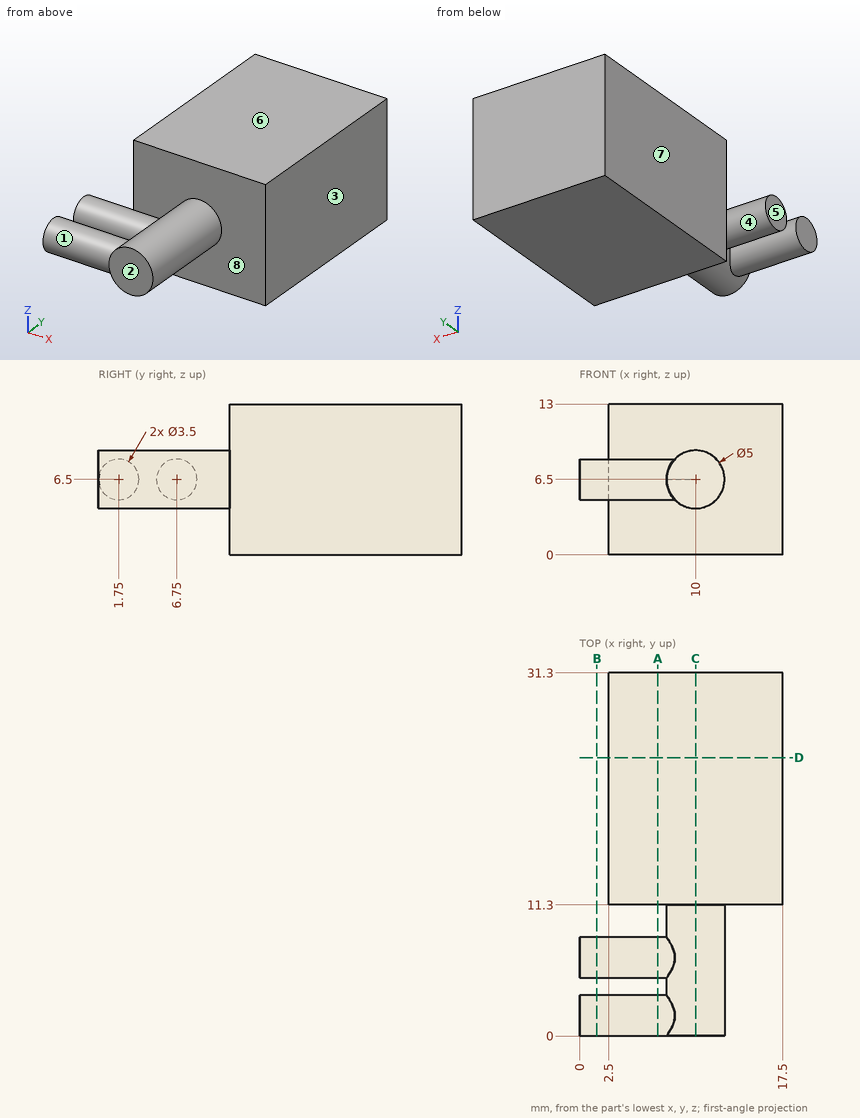
Check sheet for the drawn part. Datum: minimum x, y, z corner. Units: mm. A direction names the side the tool comes from. Round coordinates to 2 decimals unless told otherwise and drop trailing zeros. Order: outer loops, then holes, each group sorted by start corner. A loop starts at its lowest first (then second) coordinate and runs counter-clockwise, first axis right, second up. Notation, with made-up numbers: M 31,-4.5 L 59,-4.5 A24 cw 59,24.5 Z; hole C 35,70 d9. An arc over 180 degrees is marked long. Answer in a Markdown table with one row per item.
(1) Section check C-C on x = 10. Record the boundary of the cut face in (y, z), plus the area to 4 significant figures.
Findings:
| item | result |
|---|---|
| outline | M 0,4 L 11.3,4 L 11.3,0 L 31.3,0 L 31.3,13 L 11.3,13 L 11.3,9 L 0,9 Z |
| area | 316.5 mm^2 |
(2) Section check B-B on x = 1.5. Record the boundary of the cut face in (y, z), plus the area to 3 significant figures.
Findings:
| item | result |
|---|---|
| outline | C 1.75,6.5 d3.5; C 6.75,6.5 d3.5 |
| area | 19.2 mm^2 |
(3) Draft check along Y on the marked faces 1, 2 and 3. Enter one of: +Y half, -Y half, draft (parallel to the pull), parting line (faces both ways), or undercut.
Findings:
| item | result |
|---|---|
| face 1 | undercut |
| face 2 | -Y half |
| face 3 | draft |
(4) Section check A-A on x = 6.75. Record the boundary of the cut face in (y, z).
Findings:
| item | result |
|---|---|
| outline | C 1.75,6.5 d3.5; C 6.75,6.5 d3.5; M 11.3,0 L 31.3,0 L 31.3,13 L 11.3,13 Z |
(5) Material ranges on line 1 along Y through (x, z) = (12.25, 1); line 2 along X through (y, z) = (19, 11); line 3 along Z through (x, y) = (10, 9), recorded low to high. Write a range as from..to.
Findings:
| item | result |
|---|---|
| line 1 | y = 11.3..31.3 |
| line 2 | x = 2.5..17.5 |
| line 3 | z = 4..9 |
(6) Gauge pin test, flat ends, axial feed: pin 1 (4 mm diameter, centred on x = 12, y = 7, fed in from -Z); pin 2 (5 mm diameter, centred on y = 25, z = 3.5, fed in from -X). Record the tip position at first contact, or that the pin passes through.
Findings:
| item | result |
|---|---|
| pin 1 | stops at z = 4 |
| pin 2 | stops at x = 2.5 |
(7) Section check D-D on y = 24. Record the boundary of the cut face in (x, z).
Findings:
| item | result |
|---|---|
| outline | M 2.5,0 L 17.5,0 L 17.5,13 L 2.5,13 Z |
(8) Set-up check for the marked faces 4, 5, 6, 7 and 8: record each of +Z, -Z, +X, -X, +Y, -Y from which the full face is reachable in a straight line by a thin tool's end or side.
Findings:
| item | result |
|---|---|
| face 4 | -X |
| face 5 | +Z, -Z, -X, +Y, -Y |
| face 6 | +Z, +X, -X, +Y, -Y |
| face 7 | +Z, -Z, -X, +Y |
| face 8 | none |
